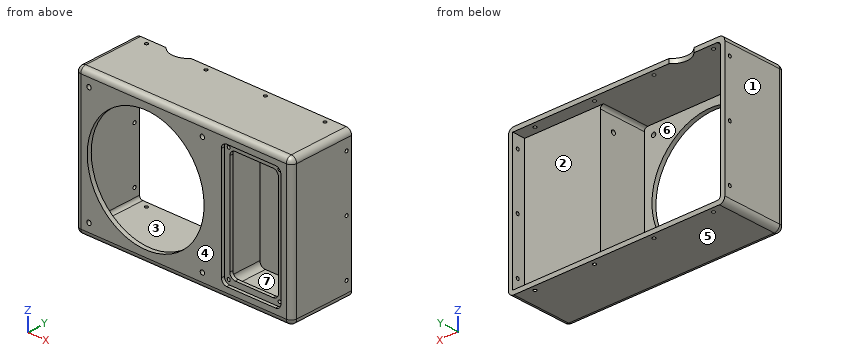
from build123d import *

# Parameters (mm, degrees)
CYLINDER010_R           = 15.2
CYLINDER010_DEPTH       = 28
CYLINDER008_R           = 1.5
CYLINDER008_DEPTH       = 210
CYLINDER008_PITCH_ANGLE = 90
CYLINDER009_R           = 1.5
CYLINDER009_DEPTH       = 210
CYLINDER009_PITCH_ANGLE = 90
CYLINDER007_R           = 1.5
CYLINDER007_DEPTH       = 210
CYLINDER007_PITCH_ANGLE = 90
CYLINDER004_R           = 1.5
CYLINDER004_DEPTH       = 140
CYLINDER006_R           = 1.5
CYLINDER006_DEPTH       = 140
CYLINDER005_R           = 1.5
CYLINDER005_DEPTH       = 140
CYLINDER003_R           = 1.5
CYLINDER003_DEPTH       = 140
SKETCH002_R             = 1.4
PAD002_DEPTH            = 25
SKETCH001_R             = 54
SKETCH001_R_2           = 2
PAD001_DEPTH            = 100
CYLINDER_R              = 2
CYLINDER_DEPTH          = 30
CYLINDER_PITCH_ANGLE    = 90
BOX008_W                = 192
BOX008_H                = 50
BOX008_DEPTH            = 122
BOX006_W                = 122
BOX006_H                = 50
BOX006_DEPTH            = 122
BOX003_W                = 66
BOX003_H                = 38
BOX003_DEPTH            = 122
BOX005_W                = 45
BOX005_H                = 40
BOX005_DEPTH            = 100
BOX004_W                = 55
BOX004_H                = 40
BOX004_DEPTH            = 110
FILLET001_R             = 5
SKETCH_W                = 200
SKETCH_H                = 60
PAD_DEPTH               = 130
FILLET_R                = 5
FILLET002_R             = 5
FILLET003_R             = 3


with BuildPart() as cylinder010:
    # Cylinder010 → Cylinder010 (new body)
    with BuildSketch(Plane(origin=(40, 70, 124), x_dir=(1, 0, 0), z_dir=(0, 0, 1))):
        Circle(CYLINDER010_R)
    extrude(amount=CYLINDER010_DEPTH)


with BuildPart() as cylinder008:
    # Cylinder008 → Cylinder008 (new body)
    with BuildSketch(Plane.XY):
        Circle(CYLINDER008_R)
    extrude(amount=CYLINDER008_DEPTH)


with BuildPart() as cylinder008_1:
    # Cylinder008 pitch: moved
    add(cylinder008.part.rotate(Axis((0, 0, 0), (0, 1, 0)), CYLINDER008_PITCH_ANGLE))


with BuildPart() as cylinder008_2:
    # Cylinder008 placement: moved
    add(cylinder008_1.part.moved(Location((-5, 0, 115))))


with BuildPart() as cylinder009:
    # Cylinder009 → Cylinder009 (new body)
    with BuildSketch(Plane.XY):
        Circle(CYLINDER009_R)
    extrude(amount=CYLINDER009_DEPTH)


with BuildPart() as cylinder009_1:
    # Cylinder009 pitch: moved
    add(cylinder009.part.rotate(Axis((0, 0, 0), (0, 1, 0)), CYLINDER009_PITCH_ANGLE))


with BuildPart() as cylinder009_2:
    # Cylinder009 placement: moved
    add(cylinder009_1.part.moved(Location((-5, 0, 65))))


with BuildPart() as fusion006:
    # Cylinder007 → Cylinder007 (new body)
    with BuildSketch(Plane.XY):
        Circle(CYLINDER007_R)
    extrude(amount=CYLINDER007_DEPTH)


with BuildPart() as fusion006_1:
    # Cylinder007 pitch: moved
    add(fusion006.part.rotate(Axis((0, 0, 0), (0, 1, 0)), CYLINDER007_PITCH_ANGLE))


with BuildPart() as fusion006_2:
    # Cylinder007 placement: moved
    add(fusion006_1.part.moved(Location((-5, 0, 15))))

    # Fusion006: union Cylinder008, Cylinder009
    add(cylinder008_2.part)
    add(cylinder009_2.part)


with BuildPart() as cylinder004:
    # Cylinder004 → Cylinder004 (new body)
    with BuildSketch(Plane(origin=(180, 0, -5), x_dir=(1, 0, 0), z_dir=(0, 0, 1))):
        Circle(CYLINDER004_R)
    extrude(amount=CYLINDER004_DEPTH)


with BuildPart() as cylinder006:
    # Cylinder006 → Cylinder006 (new body)
    with BuildSketch(Plane(origin=(125, 0, -5), x_dir=(1, 0, 0), z_dir=(0, 0, 1))):
        Circle(CYLINDER006_R)
    extrude(amount=CYLINDER006_DEPTH)


with BuildPart() as cylinder005:
    # Cylinder005 → Cylinder005 (new body)
    with BuildSketch(Plane(origin=(70, 0, -5), x_dir=(1, 0, 0), z_dir=(0, 0, 1))):
        Circle(CYLINDER005_R)
    extrude(amount=CYLINDER005_DEPTH)


with BuildPart() as fusion007:
    # Cylinder003 → Cylinder003 (new body)
    with BuildSketch(Plane(origin=(15, 0, -5), x_dir=(1, 0, 0), z_dir=(0, 0, 1))):
        Circle(CYLINDER003_R)
    extrude(amount=CYLINDER003_DEPTH)

    # Fusion005: union Cylinder004, Cylinder006, Cylinder005
    add(cylinder004.part)
    add(cylinder006.part)
    add(cylinder005.part)

    # Fusion007: union Fusion006
    add(fusion006_2.part)


with BuildPart() as fusion007_1:
    # Fusion007 placement: moved
    add(fusion007.part.moved(Location((0, 55, 0))))


with BuildPart() as pad002:
    # Sketch002 → Pad002 (new body)
    with BuildSketch(Plane.XZ.offset(10)):
        with Locations((139, 116)):
            Circle(SKETCH002_R)
        with Locations((186, 116)):
            Circle(SKETCH002_R)
        with Locations((139, 14)):
            Circle(SKETCH002_R)
        with Locations((186, 14)):
            Circle(SKETCH002_R)
    extrude(amount=-PAD002_DEPTH)


with BuildPart() as pad001:
    # Sketch001 → Pad001 (new body)
    with BuildSketch(Plane.XZ.offset(50)):
        with Locations((65, 65)):
            Circle(SKETCH001_R)
        with Locations((12.65, 117.4)):
            Circle(SKETCH001_R_2)
        with Locations((117.4, 117.4)):
            Circle(SKETCH001_R_2)
        with Locations((117.4, 12.65)):
            Circle(SKETCH001_R_2)
        with Locations((12.65, 12.65)):
            Circle(SKETCH001_R_2)
    extrude(amount=-PAD001_DEPTH)


with BuildPart() as cylinder:
    # Cylinder → Cylinder (new body)
    with BuildSketch(Plane.XY):
        Circle(CYLINDER_R)
    extrude(amount=CYLINDER_DEPTH)


with BuildPart() as cylinder_1:
    # Cylinder pitch: moved
    add(cylinder.part.rotate(Axis((0, 0, 0), (0, 1, 0)), CYLINDER_PITCH_ANGLE))


with BuildPart() as cylinder_2:
    # Cylinder placement: moved
    add(cylinder_1.part.moved(Location((120, 35, 110))))


with BuildPart() as cube008:
    # Box008 → Box008 (new body)
    with BuildSketch(Plane(origin=(4, 48, 4), x_dir=(1, 0, 0), z_dir=(0, 0, 1))):
        with Locations((96, 25)):
            Rectangle(BOX008_W, BOX008_H)
    extrude(amount=BOX008_DEPTH)


with BuildPart() as fusion003:
    # Box006 → Box006 (new body)
    with BuildSketch(Plane(origin=(4, 4, 4), x_dir=(1, 0, 0), z_dir=(0, 0, 1))):
        with Locations((61, 25)):
            Rectangle(BOX006_W, BOX006_H)
    extrude(amount=BOX006_DEPTH)

    # Fusion003: union Cube008
    add(cube008.part)


with BuildPart() as cube003:
    # Box003 → Box003 (new body)
    with BuildSketch(Plane(origin=(130, 6, 4), x_dir=(1, 0, 0), z_dir=(0, 0, 1))):
        with Locations((33, 19)):
            Rectangle(BOX003_W, BOX003_H)
    extrude(amount=BOX003_DEPTH)


with BuildPart() as cube005:
    # Box005 → Box005 (new body)
    with BuildSketch(Plane(origin=(140, -15, 15), x_dir=(1, 0, 0), z_dir=(0, 0, 1))):
        with Locations((22.5, 20)):
            Rectangle(BOX005_W, BOX005_H)
    extrude(amount=BOX005_DEPTH)


with BuildPart() as fusion002:
    # Box004 → Box004 (new body)
    with BuildSketch(Plane(origin=(135, -37, 10), x_dir=(1, 0, 0), z_dir=(0, 0, 1))):
        with Locations((27.5, 20)):
            Rectangle(BOX004_W, BOX004_H)
    extrude(amount=BOX004_DEPTH)

    # Fillet001
    fillet001_edges = [fusion002.edges().sort_by_distance(p)[0] for p in [
        (135, -17, 120),
        (135, -17, 10),
        (190, -17, 120),
        (190, -17, 10),
    ]]
    fillet(fillet001_edges, radius=FILLET001_R)

    # Fusion002: union Cube005
    add(cube005.part)


with BuildPart() as cut011:
    # Sketch → Pad (new body)
    with BuildSketch(Plane.XY):
        with Locations((100, 30)):
            Rectangle(SKETCH_W, SKETCH_H)
    extrude(amount=PAD_DEPTH)

    # Cut: cut Fusion002
    add(fusion002.part, mode=Mode.SUBTRACT)

    # Cut001: cut Cube003
    add(cube003.part, mode=Mode.SUBTRACT)

    # Fillet
    fillet_edges = [cut011.edges().sort_by_distance(p)[0] for p in [
        (140, 4.5, 115),
        (185, 4.5, 115),
        (185, 4.5, 15),
        (140, 4.5, 15),
    ]]
    fillet(fillet_edges, radius=FILLET_R)

    # Fillet002
    fillet002_edges = [cut011.edges().sort_by_distance(p)[0] for p in [
        (0, 0, 65),
        (100, 0, 0),
        (100, 0, 130),
        (200, 0, 65),
        (130, 25, 4),
        (196, 25, 4),
        (196, 25, 126),
        (130, 25, 126),
        (0, 30, 0),
        (0, 30, 130),
        (200, 30, 0),
        (200, 30, 130),
    ]]
    fillet(fillet002_edges, radius=FILLET002_R)

    # Cut002: cut Fusion003
    add(fusion003.part, mode=Mode.SUBTRACT)

    # Cut003: cut Cylinder
    add(cylinder_2.part, mode=Mode.SUBTRACT)

    # Fillet003
    fillet003_edges = [cut011.edges().sort_by_distance(p)[0] for p in [
        (126, 26, 126),
        (126, 26, 4),
        (4, 32, 126),
        (4, 32, 4),
    ]]
    fillet(fillet003_edges, radius=FILLET003_R)

    # Cut004: cut Pad001
    add(pad001.part, mode=Mode.SUBTRACT)

    # Cut005: cut Pad002
    add(pad002.part, mode=Mode.SUBTRACT)

    # Cut007: cut Fusion007
    add(fusion007_1.part, mode=Mode.SUBTRACT)

    # Cut011: cut Cylinder010
    add(cylinder010.part, mode=Mode.SUBTRACT)


solid = cut011.part
Design review of the part built by this model. Coordinates are the model's own, in mm. Face numbers are marked on the shaded views. A direction names the side the tool comes from. Give positions to 0.01 mm unless a question says otherwise; leave off trailing zeros. Loops run counter-clockwise (first coordinate to the right, second up) from the corner with the lowest first, then second, coordinate; pieces in that order, holes last. Notation, with made-up numbers: (13, -21) -> (65, -21) arc R24 cw to (65, -4) -> close; hole circle Ø7 at (15.25, 16). An arc over 180 degrees is marked (long way). One line per question, with ' | ' between items. Start each with the question number.
(1) We need section B-B (y = 18.5). State the section outline as (x, z) points, and give its area (3 significant figures).
(2) We need section C-C (x = 58). State the section outline as (y, z) points.
(3) Insertion check: P1, Ø1.8, axis at x = 15, y = 55, coming from the +Z side; P2, Ø3.5, axis at x = 152.5, y = 2, coming from the +Z side; P3, Ø12, axis at x = 22, z = 95.5, coming from the -Y side; P4, Ø1.7, axis at x = 186, z = 116, coming from the -Y side. Each pin has a flat end and moves straight along its axis. Give the tip position at first contact, or say it passes through.
(4) Draft analysis for pull direction X (two halves, no side actions). For the marked faces 1, 2, 3 and 4, state which applies: +X half, -X half, draft (parallel to the pull), parting line (faces both ways), or undercut.
(5) We need section D-D (z = 30). State the section outline as (x, y) points, and give its area (3 significant figures).
(6) We need section A-A (x = 154). State the section outline as (y, z) points, and give its area (3 significant figures).
(7) For line 1 (X direction, y = 22, z = 116.5); line 2 (Z direction, x = 186, y = 5.4); line 3 (X direction, y = 47, z = 65), list the stretches that pass through material, from the lowest coordinate up.
(8) For the marked faces 5, 6 and 7, list the 3-axis set-ups (+Z, -Z, +X, -X, +Y, -Y) from which the entire face can be reached by the end or side of a thin tool; tool diameter is ignored.
The answers:
1) outline: (0, 5) arc R5 ccw to (5, 0) -> (195, 0) arc R5 ccw to (200, 5) -> (200, 125) arc R5 ccw to (195, 130) -> (5, 130) arc R5 ccw to (0, 125) -> close; hole (4, 7) arc R3 ccw to (7, 4) -> (123, 4) arc R3 ccw to (126, 7) -> (126, 123) arc R3 ccw to (123, 126) -> (7, 126) arc R3 ccw to (4, 123) -> close; hole (130, 9) arc R5 ccw to (135, 4) -> (191, 4) arc R5 ccw to (196, 9) -> (196, 121) arc R5 ccw to (191, 126) -> (135, 126) arc R5 ccw to (130, 121) -> close | area: 3,070 mm^2
2) outline: (0, 5) arc R5 ccw to (5, 0) -> (60, 0) -> (60, 4) -> (4, 4) -> (4, 11.46) -> (0, 11.46) -> close; (0, 118.54) -> (4, 118.54) -> (4, 126) -> (60, 126) -> (60, 130) -> (5, 130) arc R5 ccw to (0, 125) -> close
3) P1: passes through | P2: stops at z = 129.84 | P3: stops at y = 0 | P4: stops at y = 44
4) face 1: -X half | face 2: undercut | face 3: undercut | face 4: draft
5) outline: (0, 5) arc R5 ccw to (5, 0) -> (23.88, 0) -> (23.88, 4) -> (4, 4) -> (4, 60) -> (0, 60) -> close; (106.12, 0) -> (135, 0) -> (135, 3) -> (140, 3) -> (140, 6) -> (130, 6) -> (130, 44) -> (196, 44) -> (196, 6) -> (185, 6) -> (185, 3) -> (190, 3) -> (190, 0) -> (195, 0) arc R5 ccw to (200, 5) -> (200, 60) -> (196, 60) -> (196, 48) -> (126, 48) -> (126, 4) -> (106.12, 4) -> close | area: 1,180 mm^2
6) outline: (0, 5) arc R5 ccw to (5, 0) -> (60, 0) -> (60, 4) -> (48, 4) -> (48, 126) -> (60, 126) -> (60, 130) -> (5, 130) arc R5 ccw to (0, 125) -> (0, 120) -> (3, 120) -> (3, 115) -> (6, 115) -> (6, 126) -> (44, 126) -> (44, 4) -> (6, 4) -> (6, 15) -> (3, 15) -> (3, 10) -> (0, 10) -> close | area: 1,060 mm^2
7) line 1: x = 0 to 4, 126 to 130, 196 to 200 | line 2: z = 0 to 12.6, 15.4 to 114.6, 117.4 to 130 | line 3: x = 0 to 4, 126 to 200
8) face 5: -Z, +X, -X, +Y, -Y | face 6: +Y | face 7: none
